```python
from build123d import *

# Parameters (mm, degrees)
F1_DEPTH = 10


# Not quite as in the source:
# - the program builds the solid bodies; features that only make, move or delete a surface that nothing else refers to are left out


with BuildPart() as f1:
    # F0 (on Top) → F1 (new body)
    with BuildSketch(Plane.XY):
        with BuildLine():
            ThreePointArc((4.2686762947, -24.6328724003), (19.1274267397, -16.0978739688), (25, 0))
            ThreePointArc((25, 0), (18.8537485405, 16.4175566383), (3.4371067222, 24.7625987606))
            ThreePointArc((3.4371067222, 24.7625987606), (-24.9964580647, -0.42081376), (4.2686762947, -24.6328724003))
        make_face()
        with BuildLine():
            ThreePointArc((110.4968080295, 19.9800743296), (95.7812936366, 14.4542523825), (89.6042668357, 0))
            ThreePointArc((89.6042668357, 0), (95.7750082208, -14.4482388602), (110.4794274519, -19.9808431728))
            ThreePointArc((110.4794274519, -19.9808431728), (124.0525056959, -13.8292586149), (129.6042668357, 0))
            ThreePointArc((129.6042668357, 0), (124.0585192182, 13.8229731991), (110.4968080295, 19.9800743296))
        make_face()
        with BuildLine():
            Line((89.6042668357, 0), (25, 0))
            ThreePointArc((25, 0), (19.1274267397, -16.0978739688), (4.2686762947, -24.6328724003))
            Line((4.2686762947, -24.6328724003), (110.4794274519, -19.9808431728))
            ThreePointArc((110.4794274519, -19.9808431728), (95.7750082208, -14.4482388602), (89.6042668357, 0))
        make_face()
        with BuildLine():
            ThreePointArc((3.4371067222, 24.7625987606), (18.8537485405, 16.4175566383), (25, 0))
            Line((25, 0), (89.6042668357, 0))
            ThreePointArc((89.6042668357, 0), (95.7812936366, 14.4542523825), (110.4968080295, 19.9800743296))
            Line((110.4968080295, 19.9800743296), (3.4371067222, 24.7625987606))
        make_face()
    extrude(amount=F1_DEPTH)


solid = f1.part
```
Geometry check sheet. Reference: the model listing, model coordinates, mm. Round coordinates to 2 decimals unless told otherwise and drop trailing zeros. Order: outer loops, then holes, each group sorted by start corner. A loop starts at its lowest first (then second) coordinate and runs counter-clockwise, first axis right, second up. Notation, with made-up numbers: (-29, 3) - (-16, 3) arc R5 cw to (-16, 10) - close; hole circle Ø7 at (42, -32.5). An arc over 180 degrees is marked (long way). Use a Markdown table: item, result. Add a question column.
1) Thickness scan on line 1 along Y through (x, z) = (-0.5, 6) (3 decimals); line 2 along X through (y, z) = (1, 0.5); line 3 along X through (y, z) = (17.5, 5.5). Record the ranges inside material, lowest first.
2) Gauge pin test, flat ends, axial feed: P1, Ø6, axis at y = 8, z = 1, coming from the +X side; P2, Ø4, axis at x = 53.5, z = 6, coming from the +Y side; P3, Ø1, axis at x = 67, z = 4.5, coming from the -Y side; P4, Ø6, axis at x = 111.5, y = -1.5, coming from the -Z side. Record the tip position at first contact, or that the pin passes through.
3) Section check C-C (y = 13). Record the cut outline in (x, z).
4) Section check A-A (z = 6.5). Record the cut outline in (x, y).
5) Section check B-B (x = 32.5). Record the cut outline in (y, z).
Established:
| question | item | result |
|---|---|---|
| 1 | line 1 | -24.995 to 24.995 |
| 1 | line 2 | -24.98 to 129.58 |
| 1 | line 3 | -17.85 to 119.29 |
| 2 | P1 | x = 128.97 |
| 2 | P2 | y = 22.62 |
| 2 | P3 | y = -21.91 |
| 2 | P4 | z = 0 |
| 3 | outline | (-21.35, 0) - (124.8, 0) - (124.8, 10) - (-21.35, 10) - close |
| 4 | outline | (3.44, 24.76) arc R25 ccw (long way) to (4.27, -24.63) - (110.48, -19.98) arc R20 ccw to (110.5, 19.98) - close |
| 5 | outline | (-23.4, 0) - (23.46, 0) - (23.46, 10) - (-23.4, 10) - close |
